Part model, mm, in its own coordinate system. Round coordinates to 2 decimals unless told otherwise and drop trailing zeros. Write each loop counter-clockwise with the first axis right and the second up, starting at its lowest first coordinate (ties: lowest second). Pieces come first, ordered by that corner, then holes. Notation, with made-up numbers: M -39.75,22 L 19.25,22 A11 ccw 19.25,30 Z; hole C 15,-9 d4. An arc over 180 degrees is marked long. Use a Markdown table: item, result. Add a question column.
1) Drop flat-ended pins along their axis: P1, Ø3, axis at x = 140, z = -65, coming from the +Y side; P2, Ø2.5, axis at y = 3, z = -79.5, coming from the +X side; P3, Ø2.5, axis at x = -154, y = 3.5, coming from the +Z side; P4, Ø1.5, axis at x = -152.5, y = 2, coming from the -Z side. Give the stop position or say it passes through.
2) Slice it at B-B on x = 91.5. Write the cut outline in (y, z), plus the area to 3 significant figures.
3) Slice it at C-C on z = -71.5. Write the cut outline in (x, y), plus the area to 3 significant figures.
4) Slice it at A-A on y = 2.5. Write the cut outline in (x, z), plus the area to 3 significant figures.
5) Wall check: probe 1 along Z at (x, y) = (-60.5, 1.35); probe 2 along Z at (x, y) = (124, 2.6); probe 3 along Z at (x, y) = (-143, 0.75). Give the ranges that are in metal, low to high.
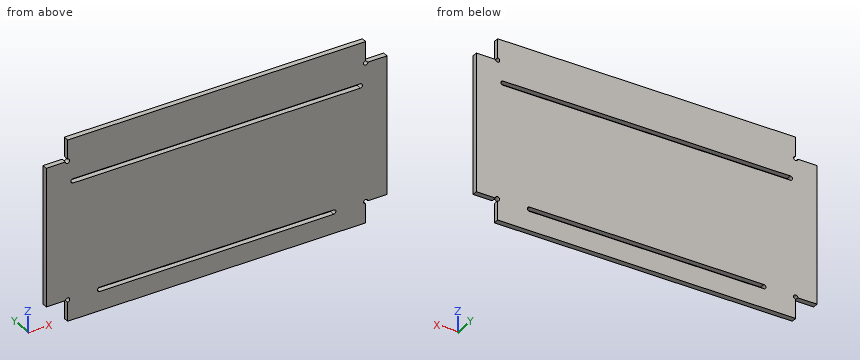
```python
from build123d import *

# Parameters (mm, degrees)
SKIZZE1_W                       = 320
SKIZZE1_H                       = 170
AUFSATZ_LINEAR_AUSTRAGEN1_DEPTH = 5
SKIZZE2_W                       = 20
SKIZZE2_H                       = 20
SCHNITT_LINEAR_AUSTRAGEN1_DEPTH = 182.245689604
SCHNITT_LINEAR_AUSTRAGEN2_DEPTH = 182.245689604
SKIZZE4_R                       = 2
SCHNITT_LINEAR_AUSTRAGEN3_DEPTH = 182.245689604


with BuildPart() as part:
    # Skizze1 → Aufsatz-Linear austragen1 (new body)
    with BuildSketch(Plane(origin=(0, 0, 0), x_dir=(1, 0, 0), z_dir=(0, 1, 0))):
        Rectangle(SKIZZE1_W, SKIZZE1_H)
    extrude(amount=AUFSATZ_LINEAR_AUSTRAGEN1_DEPTH)

    # Skizze2 → Schnitt-Linear austragen1 (cut, through all)
    with BuildSketch(Plane(origin=(0, 5, 0), x_dir=(1, 0, 0), z_dir=(0, 1, 0))):
        with Locations((-150, 75)):
            Rectangle(SKIZZE2_W, SKIZZE2_H)
        with Locations((150, 75)):
            Rectangle(SKIZZE2_W, SKIZZE2_H)
        with Locations((150, -75)):
            Rectangle(SKIZZE2_W, SKIZZE2_H)
        with Locations((-150, -75)):
            Rectangle(SKIZZE2_W, SKIZZE2_H)
    extrude(amount=-SCHNITT_LINEAR_AUSTRAGEN1_DEPTH, mode=Mode.SUBTRACT)

    # Skizze3 → Schnitt-Linear austragen2 (cut, through all)
    with BuildSketch(Plane(origin=(0, 5, 0), x_dir=(1, 0, 0), z_dir=(0, 1, 0))):
        with BuildLine():
            Line((-110, 67), (110, 67))
            ThreePointArc((110, 67), (112, 65), (110, 63))
            Line((110, 63), (-110, 63))
            ThreePointArc((-110, 63), (-112, 65), (-110, 67))
        make_face()
        with BuildLine():
            Line((-135, -43), (135, -43))
            ThreePointArc((135, -43), (137, -45), (135, -47))
            Line((135, -47), (-135, -47))
            ThreePointArc((-135, -47), (-137, -45), (-135, -43))
        make_face()
    extrude(amount=-SCHNITT_LINEAR_AUSTRAGEN2_DEPTH, mode=Mode.SUBTRACT)

    # Skizze4 → Schnitt-Linear austragen3 (cut, through all)
    with BuildSketch(Plane(origin=(0, 5, 0), x_dir=(1, 0, 0), z_dir=(0, 1, 0))):
        with Locations((-140, 65)):
            Circle(SKIZZE4_R)
        with Locations((-140, -65)):
            Circle(SKIZZE4_R)
        with Locations((140, -65)):
            Circle(SKIZZE4_R)
        with Locations((140, 65)):
            Circle(SKIZZE4_R)
    extrude(amount=-SCHNITT_LINEAR_AUSTRAGEN3_DEPTH, mode=Mode.SUBTRACT)


solid = part.part
```
Entries:
| question | item | result |
|---|---|---|
| 1 | P1 | passes through |
| 1 | P2 | stops at x = 140 |
| 1 | P3 | stops at z = 65 |
| 1 | P4 | stops at z = -65 |
| 2 | outline | M 0,-85 L 5,-85 L 5,-67 L 0,-67 Z; M 0,-63 L 5,-63 L 5,43 L 0,43 Z; M 0,47 L 5,47 L 5,85 L 0,85 Z |
| 2 | area | 810 mm^2 |
| 3 | outline | M -140,0 L 140,0 L 140,5 L -140,5 Z |
| 3 | area | 1,400 mm^2 |
| 4 | outline | M -160,-65 L -142,-65 A2 cw long -140,-67 L -140,-85 L 140,-85 L 140,-67 A2 cw long 142,-65 L 160,-65 L 160,65 L 142,65 A2 cw long 140,67 L 140,85 L -140,85 L -140,67 A2 cw long -142,65 L -160,65 Z; hole M -135,43 L 135,43 A2 ccw 135,47 L -135,47 A2 ccw Z; hole M -110,-67 L 110,-67 A2 ccw 110,-63 L -110,-63 A2 ccw Z |
| 4 | area | 50,800 mm^2 |
| 5 | probe 1 | z = -85 to -67, -63 to 43, 47 to 85 |
| 5 | probe 2 | z = -85 to 43, 47 to 85 |
| 5 | probe 3 | z = -65 to 65 |
